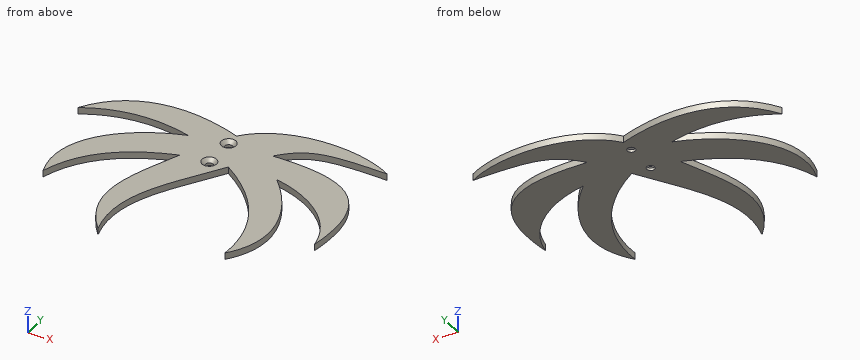
```python
from build123d import *

# Parameters (mm, degrees)
BOSS_EXTRUDE1_DEPTH                           = 3.175
CSK_FOR_6_FLAT_HEAD_MACHINE_SCREW1_AT_2_COUNT = 2
CSK_FOR_6_FLAT_HEAD_MACHINE_SCREW1_AT_2_PITCH = 15.875


with BuildPart() as part:
    # Sketch1 → Boss-Extrude1 (new body)
    with BuildSketch(Plane.XY):
        with BuildLine():
            add(Edge.make_bspline(
                [(34.931884294, 165.025383652), (48.828055098, 187.719675837), (76.45444521, 188.520066825), (100.445839981, 180.332984416), (102.354778378, 179.613312562)],
                knots=[0, 0, 0, 0, 0.389677888, 0.423902211, 0.423902211, 0.423902211, 0.423902211], degree=3))
            add(Edge.make_bspline(
                [(102.354778378, 179.613312562), (103.688252769, 181.188793447), (120.08516999, 197.822043176), (153.725104458, 196.423627733), (170.491254722, 186.467930029)],
                knots=[0.566670892, 0.566670892, 0.566670892, 0.566670892, 0.604773786, 1, 1, 1, 1], degree=3))
            add(Edge.make_bspline(
                [(122.854505464, 174.304585318), (133.217704907, 186.42088718), (141.87402844, 187.437840711), (170.491254722, 186.467930029)],
                knots=[0.652055608, 0.652055608, 0.652055608, 0.652055608, 1, 1, 1, 1], degree=3))
            add(Edge.make_bspline(
                [(122.854505464, 174.304585318), (150.100917529, 174.691970084), (179.076532886, 172.111025689), (171.253334777, 125.653941669)],
                knots=[0.582619189, 0.582619189, 0.582619189, 0.582619189, 1, 1, 1, 1], degree=3))
            add(Edge.make_bspline(
                [(133.211242061, 159.831846766), (133.979472702, 159.682774194), (151.701954736, 155.882016517), (168.618692728, 143.562281616), (171.253334777, 125.653941669)],
                knots=[0.658818977, 0.658818977, 0.658818977, 0.658818977, 0.673582965, 1, 1, 1, 1], degree=3))
            add(Edge.make_bspline(
                [(133.211242061, 159.831846766), (135.171104002, 157.821803299), (149.411618041, 141.491919338), (156.677266996, 118.334043551), (142.542206677, 101.410441691)],
                knots=[0.632989669, 0.632989669, 0.632989669, 0.632989669, 0.680758972, 1, 1, 1, 1], degree=3))
            add(Edge.make_bspline(
                [(111.168977908, 157.851131594), (130.281346763, 145.416554664), (144.493361512, 126.332685465), (142.542206677, 101.410441691)],
                knots=[0.543056126, 0.543056126, 0.543056126, 0.543056126, 1, 1, 1, 1], degree=3))
            add(Edge.make_bspline(
                [(87.881776799, 90.903091177), (80.744106998, 115.729737526), (96.501549834, 135.001149116), (109.967437477, 155.985823694), (111.168977908, 157.851131594)],
                knots=[0, 0, 0, 0, 0.464688532, 0.510268863, 0.510268863, 0.510268863, 0.510268863], degree=3))
            add(Edge.make_bspline(
                [(87.881776799, 90.903091177), (69.284973328, 112.208882094), (79.686924952, 132.536670793), (88.858930138, 154.386086423), (89.308499289, 155.455602419)],
                knots=[0, 0, 0, 0, 0.384997093, 0.404814032, 0.404814032, 0.404814032, 0.404814032], degree=3))
            add(Edge.make_bspline(
                [(46.348413822, 116.89002104), (52.796354346, 138.61615839), (70.085133937, 149.298268287), (89.308499289, 155.455602419)],
                knots=[0, 0, 0, 0, 0.378547614, 0.378547614, 0.378547614, 0.378547614], degree=3))
            add(Edge.make_bspline(
                [(46.348413822, 116.89002104), (37.891933448, 141.39657653), (59.918576266, 161.597817566), (82.928148168, 169.350328204), (84.88315803, 169.928160001)],
                knots=[0, 0, 0, 0, 0.348685432, 0.380913319, 0.380913319, 0.380913319, 0.380913319], degree=3))
            add(Edge.make_bspline(
                [(34.931884294, 165.025383652), (50.935408962, 174.180938827), (68.379973418, 174.627254849), (84.88315803, 169.928160001)],
                knots=[0, 0, 0, 0, 0.348652947, 0.348652947, 0.348652947, 0.348652947], degree=3))
        make_face()
    extrude(amount=BOSS_EXTRUDE1_DEPTH)

    # Sketch3 → CSK for #6 Flat Head Machine Screw1 (revolve, cut)
    with BuildSketch(Plane(origin=(102.354778378, 173.263312562, 3.175), x_dir=(0, -1, 0), z_dir=(1, 0, 0))):
        Polygon((0, 0), (0, 3.175), (1.89865, 3.175), (1.89865, 1.891953401), (3.5433, 0), align=None)
    csk_for_6_flat_head_machine_screw1 = revolve(axis=Axis((102.354778378, 173.263312562, 9.525), (0, 0, -1)), mode=Mode.SUBTRACT)

    # CSK for #6 Flat Head Machine Screw1 at 2: CSK for #6 Flat Head Machine Screw1 ×2
    with Locations(*[(0, -i * CSK_FOR_6_FLAT_HEAD_MACHINE_SCREW1_AT_2_PITCH, 0) for i in range(1, CSK_FOR_6_FLAT_HEAD_MACHINE_SCREW1_AT_2_COUNT)]):
        add(csk_for_6_flat_head_machine_screw1, mode=Mode.SUBTRACT)


solid = part.part
```
For this review, take the finished solid that the model builds, in its own axes (mm). Round coordinates to 2 decimals unless told otherwise and drop trailing zeros. One line per item, written item: value. Start each with the question number.
(1) We need section A-A (z = 2.15). Count the separate pieces of the cut face and the enclosed holes in it, and give its area (3 significant figures).
(2) Insertion check: pin 1 (1 mm diameter, centred on x = 64, z = 0.5, fed in from -Y) (3 decimals); pin 2 (1 mm diameter, centred on y = 145, z = 2.5, fed in from +X). Each pin has a flat end and moves straight along its axis. Give the tip position at first contact, or say it passes through.
(3) Wall thickness on line 1 (Y direction, x = 104, z = 3.05); line 2 (Y direction, x = 145, z = 2.3); line 3 (X direction, y = 119, z = 1.65): over which ranges is each line inside the solid? List them lowest first.
Result:
1. separate pieces: 1
1. enclosed holes: 2
1. area: 5,010 mm²
2. pin 1: y = 142.385
2. pin 2: x = 172.36
3. line 1: 146.93 to 154.37, 160.4 to 170.25, 176.28 to 181.44
3. line 2: 104.68 to 143.85, 156.23 to 173.09, 186.18 to 193.88
3. line 3: 45.69 to 47.02, 77.4 to 88.53, 141.15 to 150.41
